Verification items for this drawing (mm, ordinates from the low corner). A direction names the side the tool comes from. Round coordinates to 2 decimals unless told otherwise and drop trailing zeros. Order: outer loops, then holes, each group sorted by start corner. A loop starts at its lowest first (then second) coordinate and runs counter-clockwise, first axis right, second up. Notation, with made-up numbers: M 55,-28 L 66,-28 A31 cw 66,-4 Z; hole C 73,24.25 d1. An arc over 180 degrees is marked long. Use CSV: the item, a comma, the result in double quotes. Start each with the question number.
Q1. Sectioned sample at D-D (z = 14). Enter the section's corners in (x, y).
Q2. Sectioned sample at C-C (x = 6.35). Enter the section's corners in (y, z).
Q3. Scan lines: line 1 (Z direction, x = 6.35, y = 49); line 2 (X direction, y = 48.25, z = 20.32); line 3 (Y direction, x = 23.25, z = 20.32) (1 decimal). Record each from-to range of solid material in increasing order.
Q4. Sectioned sample at A-A (z = 20.32). State how many separate pieces and enclosed holes the cut face has, and give its area (3 significant figures).
Q5. Set-up check for the marked faces 1 and 2: record each of +Z, -Z, +X, -X, +Y, -Y from which the full face is reachable in a straight line by a thin tool's end or side.
Q6. Gauge pin test, flat ends, axial feed: pin 1 Ø4 at (y, z) = (11.43, 20.32) entering from +X; pin 2 Ø15 at (x, z) = (9, 17) entering from -Y; pin 3 Ø1 at (y, z) = (34, 7) entering from -X; pin 4 Ø12 at (y, z) = (18.5, 19.5) entering from -X. Record the tip position at first contact, or that the pin passes through.
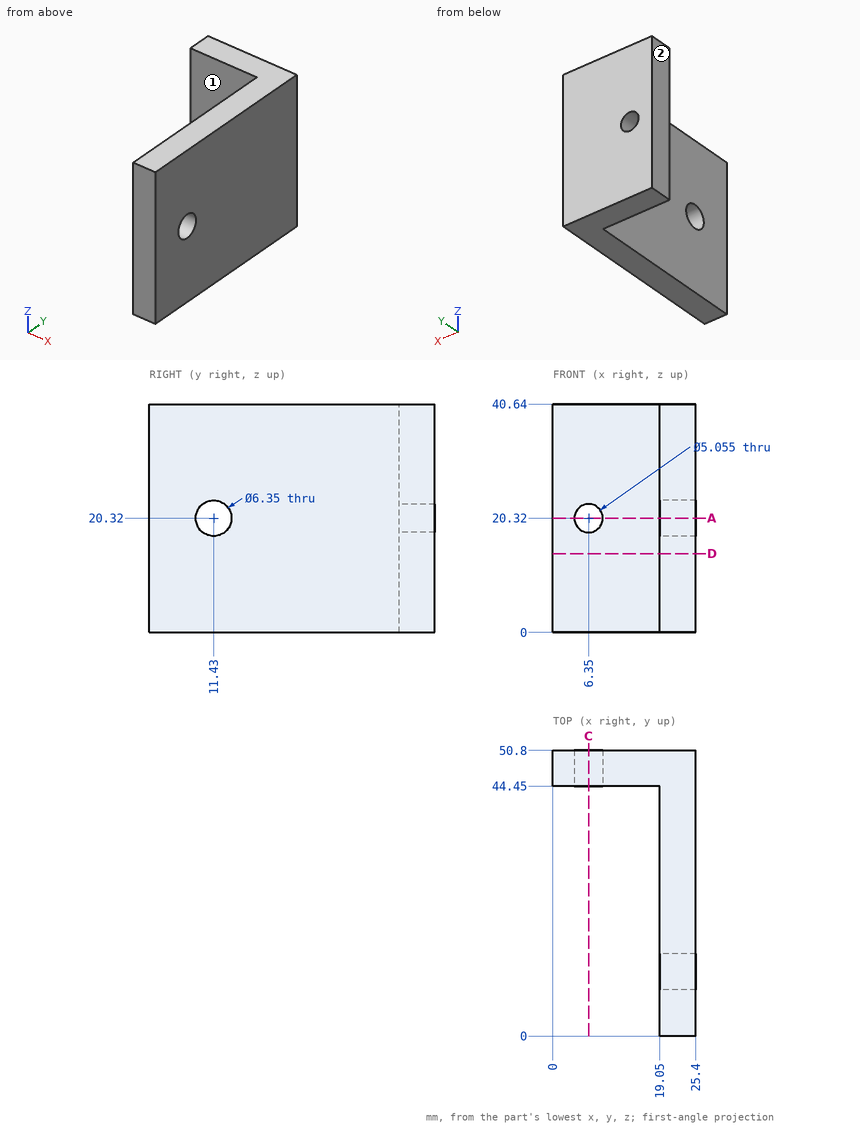
Verdict:
1,outline,"M 0,44.45 L 19.05,44.45 L 19.05,0 L 25.4,0 L 25.4,50.8 L 0,50.8 Z"
2,outline,"M 44.45,0 L 50.8,0 L 50.8,17.79 L 44.45,17.79 Z; M 44.45,22.85 L 50.8,22.85 L 50.8,40.64 L 44.45,40.64 Z"
3,line 1,"z = 0 to 17.79, 22.85 to 40.64"
3,line 2,"x = 0 to 3.82, 8.88 to 25.4"
3,line 3,"y = 0 to 8.3, 14.6 to 50.8"
4,separate pieces,"3"
4,enclosed holes,"0"
4,area,"371 mm²"
5,face 1,"+Z, -Z, -X, -Y"
5,face 2,"+Z, -Z, -X, +Y, -Y"
6,pin 1,"passes through"
6,pin 2,"stops at y = 44.45"
6,pin 3,"stops at x = 19.05"
6,pin 4,"stops at x = 19.05"
